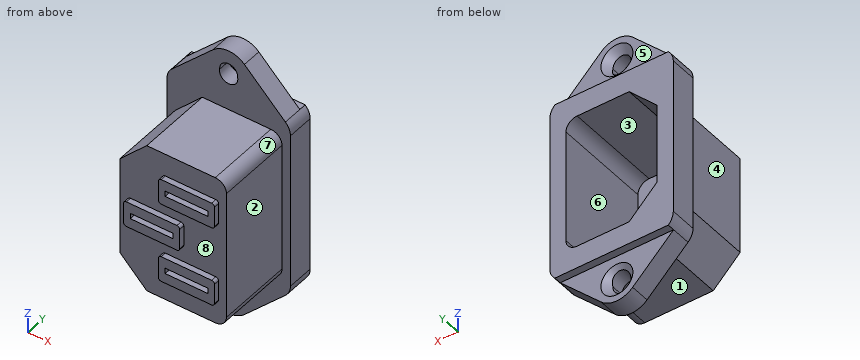
Autodesk Inventor part; units mm, degrees
ref_plane "YZ Plane" through (0, 0, 0) normal (1, 0, 0) x (0, 1, 0)
ref_plane "XZ Plane" through (0, 0, 0) normal (0, 1, 0) x (-1, 0, 0)
ref_plane "XY Plane" through (0, 0, 0) normal (0, 0, 1) x (1, 0, 0)
sketch "Sketch1" plane through (0, 0, 0) normal (0, 1, 0) x (-1, 0, 0)
  arc A0 (2.8034, 23.3533) -> (-2.8034, 23.3533) centre (0, 20.5) ccw
  line L0 (-11, 14.0418) -> (-11, 0)
  line L1 (11, 14.0418) -> (11, 0)
  line L2 (11, 0) -> (-11, 0)
  line L3 (10.1025, 16.1818) -> (2.8034, 23.3533)
  line L4 (-10.1025, 16.1818) -> (-2.8034, 23.3533)
  arc A1 (11, 14.0418) -> (10.1025, 16.1818) centre (8, 14.0418) ccw
  arc A2 (-10.1025, 16.1818) -> (-11, 14.0418) centre (-8, 14.0418) ccw
  arc A3 (-2.8034, -23.3533) -> (2.8034, -23.3533) centre (0, -20.5) ccw
  line L5 (-11, -14.0418) -> (-11, 0)
  line L6 (11, -14.0418) -> (11, 0)
  line L7 (10.1025, -16.1818) -> (2.8034, -23.3533)
  line L8 (-10.1025, -16.1818) -> (-2.8034, -23.3533)
  arc A4 (10.1025, -16.1818) -> (11, -14.0418) centre (8, -14.0418) ccw
  arc A5 (-11, -14.0418) -> (-10.1025, -16.1818) centre (-8, -14.0418) ccw
  point P0 (0, 0)
  point P1 (11, 15.3)
  point P2 (-11, 15.3)
  point P3 (11, -15.3)
  point P4 (-11, -15.3)
  dimension "d0" = 0
  dimension "d1" = 22
  dimension "d2" = 11
  dimension "d3" = 8
  dimension "d4" = 15.3
  dimension "d5" = 0
  dimension "d6" = 15.3
  dimension "d7" = 20.5
  dimension "d8" = 3
extrude "Extrusion1" add sketch "Sketch1" along normal blind 4.8
sketch "Sketch2" plane through (0, 4.8, 0) normal (0, 1, 0) x (1, 0, 0)
  line L0 (-10.1025, -16.1818) -> (-2.8034, -23.3533)
  line L1 (2.8034, -23.3533) -> (10.1025, -16.1818)
  line L2 (-10.1025, -16.1818) -> (10.1025, -16.1818)
  line L3 (-2.8034, 23.3533) -> (-10.1025, 16.1818)
  line L4 (10.1025, 16.1818) -> (2.8034, 23.3533)
  line L5 (-10.1025, 16.1818) -> (10.1025, 16.1818)
  arc A0 (-2.8034, -23.3533) -> (2.8034, -23.3533) centre (0, -20.5) ccw
  arc A1 (2.8034, 23.3533) -> (-2.8034, 23.3533) centre (0, 20.5) ccw
  point P0 (0, 0)
extrude "Extrusion2" cut sketch "Sketch2" against normal blind 1.3
sketch "Sketch3" plane through (0, 3.5, 0) normal (0, 1, 0) x (1, 0, 0)
  arc A0 (-2.8034, -23.3533) -> (2.8034, -23.3533) centre (0, -20.5) ccw
  point P0 (0, 0)
  point P1 (0, 20.5)
hole "Hole1" at (0, 3.5, 20.5) at (0, 3.5, -20.5) direction (0, -1, 0) diameter 3.2 depth 8 tip angle 118 countersink diameter 5.7 countersink angle 90
sketch "Sketch5" plane through (0, 0, 0) normal (0, -1, 0) x (1, 0, 0)
  line L0 (7.5, -13.55) -> (-4.7, -13.55)
  line L1 (-9.5, -8.75) -> (-9.5, 8.75)
  line L2 (-4.7, 13.55) -> (7.5, 13.55)
  line L3 (9.5, 11.55) -> (9.5, -11.55)
  line L4 (9.5, -13.55) -> (-9.5, 13.55) construction
  line L5 (-9.5, -13.55) -> (9.5, 13.55) construction
  line L6 (-9.5, -8.75) -> (-4.7, -13.55)
  line L7 (-9.5, 8.75) -> (-4.7, 13.55)
  arc A0 (7.5, -13.55) -> (9.5, -11.55) centre (7.5, -11.55) ccw
  arc A1 (9.5, 11.55) -> (7.5, 13.55) centre (7.5, 11.55) ccw
  point P0 (0, 0)
  dimension "d20" = 4.8
  dimension "d21" = 4.8
  dimension "d22" = 4.8
  dimension "d23" = 4.8
  dimension "d24" = 19
  dimension "d25" = 2
  dimension "d26" = 27.1
extrude "Extrusion3" add sketch "Sketch5" along normal blind 13.5
sketch "Sketch6" plane through (0, 4.8, 0) normal (0, 1, 0) x (1, 0, 0)
  line L0 (6.13, -12.15) -> (-3.13, -12.15)
  line L1 (-8.13, -7.15) -> (-8.13, 7.15)
  line L2 (-3.13, 12.15) -> (6.13, 12.15)
  line L3 (8.13, 10.15) -> (8.13, -10.15)
  line L4 (8.13, -12.15) -> (-8.13, 12.15) construction
  line L5 (-8.13, -12.15) -> (8.13, 12.15) construction
  arc A0 (6.13, -12.15) -> (8.13, -10.15) centre (6.13, -10.15) ccw
  arc A1 (8.13, 10.15) -> (6.13, 12.15) centre (6.13, 10.15) ccw
  line L6 (-8.13, -7.15) -> (-3.13, -12.15)
  line L7 (-8.13, 7.15) -> (-3.13, 12.15)
  point P0 (0, 0)
  dimension "d29" = 2
  dimension "d30" = 24.3
  dimension "d31" = 16.26
  dimension "d32" = 5
  dimension "d33" = 45
  dimension "d34" = 5
  dimension "d35" = 45
extrude "Extrusion4" cut sketch "Sketch6" against normal blind 17.5
sketch "Sketch7" plane through (0, -13.5, 0) normal (0, -1, 0) x (1, 0, 0)
  line L0 (1.4, -2.3) -> (-7.6, -2.3)
  line L1 (-8.1, -1.8) -> (-8.1, 1.8)
  line L2 (-7.6, 2.3) -> (1.4, 2.3)
  line L3 (1.9, 1.8) -> (1.9, -1.8)
  line L4 (1.9, -2.3) -> (-8.1, 2.3) construction
  line L5 (-8.1, -2.3) -> (1.9, 2.3) construction
  line L6 (7.6, -9.5) -> (-1.4, -9.5)
  line L7 (-1.9, -9) -> (-1.9, -5.4)
  line L8 (-1.4, -4.9) -> (7.6, -4.9)
  line L9 (8.1, -5.4) -> (8.1, -9)
  line L10 (8.1, -9.5) -> (-1.9, -4.9) construction
  line L11 (-1.9, -9.5) -> (8.1, -4.9) construction
  line L12 (-9.5, -8.75) -> (-4.7, -13.55)
  line L13 (-4.7, -13.55) -> (7.5, -13.55)
  arc A0 (7.5, -13.55) -> (9.5, -11.55) centre (7.5, -11.55) ccw
  line L14 (9.5, -11.55) -> (9.5, 11.55)
  arc A1 (9.5, 11.55) -> (7.5, 13.55) centre (7.5, 11.55) ccw
  line L15 (7.5, 13.55) -> (-4.7, 13.55)
  line L16 (-4.7, 13.55) -> (-9.5, 8.75)
  line L17 (-9.5, 8.75) -> (-9.5, -8.75)
  line L18 (-9.5, 0) -> (9.5, 0)
  arc A2 (-8.1, -1.8) -> (-7.6, -2.3) centre (-7.6, -1.8) ccw
  arc A3 (-7.6, 2.3) -> (-8.1, 1.8) centre (-7.6, 1.8) ccw
  arc A4 (1.9, 1.8) -> (1.4, 2.3) centre (1.4, 1.8) ccw
  arc A5 (1.4, -2.3) -> (1.9, -1.8) centre (1.4, -1.8) ccw
  arc A6 (-1.4, -4.9) -> (-1.9, -5.4) centre (-1.4, -5.4) ccw
  arc A7 (8.1, -5.4) -> (7.6, -4.9) centre (7.6, -5.4) ccw
  arc A8 (7.6, -9.5) -> (8.1, -9) centre (7.6, -9) ccw
  arc A9 (-1.9, -9) -> (-1.4, -9.5) centre (-1.4, -9) ccw
  line L19 (7.6, 9.5) -> (-1.4, 9.5)
  line L20 (-1.9, 9) -> (-1.9, 5.4)
  line L21 (-1.4, 4.9) -> (7.6, 4.9)
  line L22 (8.1, 5.4) -> (8.1, 9)
  line L23 (8.1, 9.5) -> (-1.9, 4.9) construction
  line L24 (-1.9, 9.5) -> (8.1, 4.9) construction
  arc A10 (-1.9, 5.4) -> (-1.4, 4.9) centre (-1.4, 5.4) ccw
  arc A11 (7.6, 4.9) -> (8.1, 5.4) centre (7.6, 5.4) ccw
  arc A12 (8.1, 9) -> (7.6, 9.5) centre (7.6, 9) ccw
  arc A13 (-1.4, 9.5) -> (-1.9, 9) centre (-1.4, 9) ccw
  point P0 (0, 0)
  point P1 (-3.1, 0)
  point P2 (3.1, -7.2)
  point P3 (3.1, 7.2)
  dimension "d38" = 10
  dimension "d39" = 4.6
  dimension "d40" = 2.6
  dimension "d41" = 10
  dimension "d42" = 4.6
  dimension "d43" = 0.5
  dimension "d44" = 1.4
  dimension "d45" = 1.4
extrude "Extrusion5" add sketch "Sketch7" along normal blind 1 contours L0 A2 L1 L18 L3 A5 | L18 L1 A3 L2 A4 L3 | L6 A9 L7 A6 L8 A7 L9 A8 | A12 L22 A11 L21 A10 L20 A13 L19
sketch "Sketch8" plane through (0, -14.5, 0) normal (0, -1, 0) x (1, 0, 0)
  line L0 (-7.6, -2.3) -> (1.4, -2.3)
  arc A0 (1.4, -2.3) -> (1.9, -1.8) centre (1.4, -1.8) ccw
  line L1 (1.9, -1.8) -> (1.9, 1.8)
  arc A1 (1.9, 1.8) -> (1.4, 2.3) centre (1.4, 1.8) ccw
  line L2 (1.4, 2.3) -> (-7.6, 2.3)
  arc A2 (-7.6, 2.3) -> (-8.1, 1.8) centre (-7.6, 1.8) ccw
  line L3 (-8.1, 1.8) -> (-8.1, -1.8)
  arc A3 (-8.1, -1.8) -> (-7.6, -2.3) centre (-7.6, -1.8) ccw
  line L4 (7.6, -4.9) -> (-1.4, -4.9)
  arc A4 (-1.4, -4.9) -> (-1.9, -5.4) centre (-1.4, -5.4) ccw
  line L5 (-1.9, -5.4) -> (-1.9, -9)
  arc A5 (-1.9, -9) -> (-1.4, -9.5) centre (-1.4, -9) ccw
  line L6 (-1.4, -9.5) -> (7.6, -9.5)
  arc A6 (7.6, -9.5) -> (8.1, -9) centre (7.6, -9) ccw
  line L7 (8.1, -9) -> (8.1, -5.4)
  arc A7 (8.1, -5.4) -> (7.6, -4.9) centre (7.6, -5.4) ccw
  line L8 (-1.9, 9) -> (-1.9, 5.4)
  arc A8 (-1.9, 5.4) -> (-1.4, 4.9) centre (-1.4, 5.4) ccw
  line L9 (-1.4, 4.9) -> (7.6, 4.9)
  arc A9 (7.6, 4.9) -> (8.1, 5.4) centre (7.6, 5.4) ccw
  line L10 (8.1, 5.4) -> (8.1, 9)
  arc A10 (8.1, 9) -> (7.6, 9.5) centre (7.6, 9) ccw
  line L11 (7.6, 9.5) -> (-1.4, 9.5)
  arc A11 (-1.4, 9.5) -> (-1.9, 9) centre (-1.4, 9) ccw
  line L12 (-8.1, 1.8) -> (-8.1, -1.8)
  line L13 (-8.1, 0) -> (1.9, 0)
  line L14 (-7.6, -2.3) -> (1.4, -2.3)
  line L15 (-3.1, -2.3) -> (-3.1, 2.3)
  line L16 (-1.9, -5.4) -> (-1.9, -9)
  line L17 (-1.9, -7.2) -> (8.1, -7.2)
  line L18 (7.6, -9.5) -> (-1.4, -9.5)
  line L19 (3.1, -9.5) -> (3.1, -4.9)
  line L20 (7.6, -4.9) -> (-1.4, -4.9)
  line L21 (3.1, 4.9) -> (3.1, 9.5)
  line L22 (-1.9, 9) -> (-1.9, 5.4)
  line L23 (-1.9, 7.2) -> (8.1, 7.2)
  line L24 (6.9, -7.7) -> (-0.7, -7.7)
  line L25 (-0.7, -7.7) -> (-0.7, -6.7)
  line L26 (-0.7, -6.7) -> (6.9, -6.7)
  line L27 (6.9, -6.7) -> (6.9, -7.7)
  line L28 (6.9, -7.7) -> (-0.7, -6.7) construction
  line L29 (-0.7, -7.7) -> (6.9, -6.7) construction
  line L30 (0.7, -0.5) -> (-6.9, -0.5)
  line L31 (-6.9, -0.5) -> (-6.9, 0.5)
  line L32 (-6.9, 0.5) -> (0.7, 0.5)
  line L33 (0.7, 0.5) -> (0.7, -0.5)
  line L34 (0.7, -0.5) -> (-6.9, 0.5) construction
  line L35 (-6.9, -0.5) -> (0.7, 0.5) construction
  line L36 (6.9, 6.7) -> (-0.7, 6.7)
  line L37 (-0.7, 6.7) -> (-0.7, 7.7)
  line L38 (-0.7, 7.7) -> (6.9, 7.7)
  line L39 (6.9, 7.7) -> (6.9, 6.7)
  line L40 (6.9, 6.7) -> (-0.7, 7.7) construction
  line L41 (-0.7, 6.7) -> (6.9, 7.7) construction
  point P0 (0, 0)
  point P1 (3.1, -7.2)
  point P2 (-3.1, 0)
  point P3 (3.1, 7.2)
  dimension "d48" = 7.6
  dimension "d49" = 7.6
  dimension "d50" = 7.6
  dimension "d52" = 1
  dimension "d53" = 1
  dimension "d54" = 1
extrude "Extrusion6" cut sketch "Sketch8" against normal through all contours L30 L31 L13 L15 | L15 L13 L33 L30 | L15 L32 L33 L13 | L13 L31 L32 L15 | L26 L27 L17 L19 | L19 L17 L25 L26 | L19 L24 L25 L17 | L17 L27 L24 L19 | L37 L38 L21 L23 | L23 L21 L36 L37 | L23 L39 L36 L21 | L21 L38 L39 L23
sketch "Sketch9" plane through (0, 3.5, 0) normal (0, 1, 0) x (1, 0, 0)
  circle A0 centre (0, 20.5) radius 1.6
  circle A1 centre (0, 20.5) radius 0.2629
  circle A2 centre (0, 20) radius 1.625
  line L0 (0, 20) -> (0, -20)
  circle A3 centre (0, -20) radius 1.625
  point P0 (0, 0)
  point P1 (-1.591, 20.3306)
  point P2 (1.591, 20.3306)
  dimension "d57" = 3.25
  dimension "d58" = 0.5
  dimension "d61" = 40
  dimension "d62" = 3.25
extrude "Extrusion7" cut sketch "Sketch9" against normal blind 10 contours A3 | A0 L0 A2 | A2 L0 A0
equation "\"d21\" = d20"
equation "\"d22\" = d20"
equation "\"d23\" = d22"
equation "\"d34\" = d32"
equation "\"d35\" = d33"
equation "\"d42\" = d39"
equation "\"d49\" = d48"
equation "\"d50\" = d48"
equation "\"d53\" = d52"
equation "\"d54\" = d52"
properties part number "PlugFemeaTomada" material "Plastic, Opaque Black"
Can you work these out from the model? Positions are in its coordinate system, mm. Face numbers are marked on the shaded views. A direction names the side the tool comes from. Round coordinates to 2 decimals unless told otherwise and drop trailing zeros. Write each loop counter-clockwise with the first axis right and the second up, starting at its lowest first coordinate (ties: lowest second). Pieces come first, ordered by that corner, then holes. Notation, with made-up numbers: (4.5, 9) -> (44.5, 9) arc R24 ccw to (44.5, 35) -> close; hole circle Ø4 at (22.25, -10.5). An arc over 180 degrees is marked (long way). Use one line per item in the form item = value. Start each with the question number.
Q1. If I drill on probe 1 along X at (y, z) = (-2.25, -1); probe 2 along Z at (x, y) = (4, -11.75); probe 3 along X at (y, z) = (2, -2.5), over which ranges is the centre line in solid material (lowest first)? Write a range as [from, to].
Q2. Imagine slicing it at D-D (x = 0). Count the separate pieces of the cut face and the enclosed holes in it, then the cut area to 3 significant figures.
Q3. I'm going to push flat-ended pins straight in: P1, Ø5, axis at y = -8, z = 1.5, coming from the -X side; P2, Ø8, axis at x = 7, y = -0.5, coming from the -Z side; P3, Ø5, axis at x = 5, y = -9.5, coming from the -Z side. Where does each tip first touch, or does it pass through?
Q4. Imagine slicing it at A-A (y = -9.25). Please give me the cut outline in (x, z), then the cut area to 3 significant figures.
Q5. Imagine slicing it at B-B (z = -6). Please give me the cut outline in (x, y), then the cut area to 4 significant figures.
Q6. Which directions (+Z, -Z, +X, -X, +Y, -Y) give clear straight access to the entire face, cutting with the end or side of a thin tool? Please do the marked faces 4, 5, 6, 7 and 8.
Q7. Imagine slicing it at C-C (x = -6.25). Please give me the cut outline in (y, z), then the cut area to 3 significant figures.
Q8. We'd pull the mould along Z, two halves only. Please class the marked faces 1, 2 and 3: +Z half, -Z half, draft (parallel to the pull), parting line (faces both ways), or undercut.
Worked out:
q1.probe_1 = [-9.5, -8.13], [8.13, 9.5]
q1.probe_2 = [-13.55, -12.15], [12.15, 13.55]
q1.probe_3 = [-11, -8.13], [8.13, 11]
q2.separate_pieces = 6
q2.enclosed_holes = 0
q2.area = 134 mm^2
q3.P1 = -9.5
q3.P2 = -23.13
q3.P3 = -13.55
q4.outline = (-9.5, -8.75) -> (-4.7, -13.55) -> (7.5, -13.55) arc R2 ccw to (9.5, -11.55) -> (9.5, 11.55) arc R2 ccw to (7.5, 13.55) -> (-4.7, 13.55) -> (-9.5, 8.75) -> close; hole (-8.13, -7.15) -> (-3.13, -12.15) -> (6.13, -12.15) arc R2 ccw to (8.13, -10.15) -> (8.13, 10.15) arc R2 ccw to (6.13, 12.15) -> (-3.13, 12.15) -> (-8.13, 7.15) -> close
q4.area = 122 mm^2
q5.outline = (-11, 0) -> (-9.5, 0) -> (-9.5, -13.5) -> (-1.9, -13.5) -> (-1.9, -14.5) -> (8.1, -14.5) -> (8.1, -13.5) -> (9.5, -13.5) -> (9.5, 0) -> (11, 0) -> (11, 4.8) -> (8.13, 4.8) -> (8.13, -12.7) -> (-8.13, -12.7) -> (-8.13, 4.8) -> (-11, 4.8) -> close
q5.area = 87.55 mm^2
q6.face_4 = +Z, -Z, -X, -Y
q6.face_5 = +Z, +X, -X, +Y
q6.face_6 = +Y
q6.face_7 = +Z, +X, -Y
q6.face_8 = -Y
q7.outline = (-14.5, -2.3) -> (-13.5, -2.3) -> (-13.5, -12) -> (0, -12) -> (0, -19.97) -> (3.5, -19.97) -> (3.5, -16.18) -> (4.8, -16.18) -> (4.8, -9.03) -> (-12.7, -9.03) -> (-12.7, -0.5) -> (-14.5, -0.5) -> close; (-14.5, 0.5) -> (-12.7, 0.5) -> (-12.7, 9.03) -> (4.8, 9.03) -> (4.8, 16.18) -> (3.5, 16.18) -> (3.5, 19.97) -> (0, 19.97) -> (0, 12) -> (-13.5, 12) -> (-13.5, 2.3) -> (-14.5, 2.3) -> close
q7.area = 193 mm^2
q8.face_1 = -Z half
q8.face_2 = draft
q8.face_3 = undercut
